For this review, take the finished solid that the model builds, in its own axes (mm). Face numbers are marked on the shaded views. A direction names the side the tool comes from. Coordinates: 2 decimals unless noted, no trailing zeros. Loops run counter-clockwise (first coordinate to the right, second up) from the corner with the lowest first, then second, coordinate; pieces in that order, holes last. Notation, with made-up numbers: (80, 83.5) - (85, 83.5) arc R30 ccw to (85, 118.5) - close; hole circle Ø2 at (47, 61). An arc over 180 degrees is marked (long way). Answer as a JSON object with one key per item and string values. Group by question number.
Item 1: We need section D-D (y = 0.5). Give the boundary of the cut face in (x, z).
Item 2: We need section A-A (y = -12). Give the boundary of the cut face in (x, z).
Item 3: We need section B-B (x = 30.5). Give the boundary of the cut face in (y, z), then the cut area to 3 significant figures.
Item 4: To check wall thickness, follow line 1 (Z direction, x = 13, y = 0.75); line 2 (X direction, y = 0, z = 18); line 3 (Y direction, x = 2, z = 17.5). State the ranges of each line that lie inside material, in increasing order.
Item 5: We need section C-C (z = 24.5). Give the boundary of the cut face in (x, y), then the cut area to 3 significant figures.
Item 6: Clearance check with flat-ended pins moving along their axes: pin 1 (2.5 mm diameter, centred on x = 10.5, z = 1.5, fed in from -Y); pin 2 (1 mm diameter, centred on x = 0, y = 0, fed in from +Z); pin 3 (2.5 mm diameter, centred on y = -6.5, z = 1.5, fed in from -X). State where each tip first meets the part, or that it passes through.
Item 7: Tool access review of the marked faces 1 and 2: name each direction out of +Z, -Z, +X, -X, +Y, -Y from which nothing blocks a thin tool from reaching the whole face with its end or side.
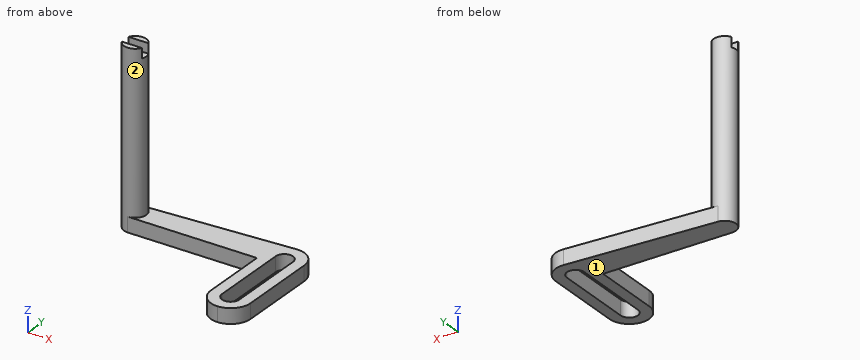
from build123d import *

# Parameters (mm, degrees)
EXTRUDE_1_DEPTH     = 3
SKETCH_1_3_R        = 2.25
EXTRUDE_2_DEPTH     = 35
SKETCH_2_W          = 5
SKETCH_2_H          = 2
CUT_EXTRUDE_1_DEPTH = 2
FILLET_1_R          = 4


with BuildPart() as part:
    # 草图1 → 凸台-拉伸1 (new body)
    with BuildSketch(Plane.XY):
        with BuildLine():
            Line((29.766666667, 3.993188645), (-0.13125, 2.246168613))
            ThreePointArc((-0.13125, 2.246168613), (-2.249041949, -0.065652955), (0, -2.25))
            Line((0, -2.25), (26, -2.25))
            Line((26, -2.25), (26, -20))
            Line((26, -20), (34, -20))
            Line((34, -20), (34, 0))
            ThreePointArc((34, 0), (32.744691847, 2.909753712), (29.766666667, 3.993188645))
        make_face()
        with BuildLine():
            Line((28.25, -16), (28.25, 0))
            ThreePointArc((28.25, 0), (30, 1.75), (31.75, 0))
            Line((31.75, 0), (31.75, -16))
            ThreePointArc((31.75, -16), (30, -17.75), (28.25, -16))
        make_face(mode=Mode.SUBTRACT)
    extrude(amount=EXTRUDE_1_DEPTH)

    # 草图1<3> → 凸台-拉伸2 (add)
    with BuildSketch(Plane.XY):
        with Locations(Location((0, 0, 0), (0, 0, 93.344152204))):
            Circle(SKETCH_1_3_R)
    extrude(amount=EXTRUDE_2_DEPTH)

    # 草图2 → 切除-拉伸1 (cut)
    with BuildSketch(Plane.XY.offset(35)):
        Rectangle(SKETCH_2_W, SKETCH_2_H)
    extrude(amount=-CUT_EXTRUDE_1_DEPTH, mode=Mode.SUBTRACT)

    # 圆角1
    fillet_1_edges = [part.edges().sort_by_distance(p)[0] for p in [
        (26, -20, 1.5),
        (34, -20, 1.5),
    ]]
    fillet(fillet_1_edges, radius=FILLET_1_R - 0.0001)  # a hair under: the kernel refuses the full size


solid = part.part
Check sheet entries:
{
 "1": {"outline": "(-2.19, 0) - (28.32, 0) - (28.32, 3) - (2.19, 3) - (2.19, 33) - (-2.19, 33) - close; (31.68, 0) - (33.97, 0) - (33.97, 3) - (31.68, 3) - close"},
 "2": {"outline": "(26, 0) - (28.25, 0) - (28.25, 3) - (26, 3) - close; (31.75, 0) - (34, 0) - (34, 3) - (31.75, 3) - close"},
 "3": {"outline": "(-19.97, 0) - (-17.68, 0) - (-17.68, 3) - (-19.97, 3) - close; (1.68, 0) - (3.97, 0) - (3.97, 3) - (1.68, 3) - close", "area": "13.7 mm2"},
 "4": {"line 1": "z = 0 to 3", "line 2": "x = -2.25 to 2.25", "line 3": "y = -1.03 to 1.03"},
 "5": {"outline": "circle Ø4.5 at (0, 0)", "area": "15.9 mm2"},
 "6": {"pin 1": "stops at y = -2.25", "pin 2": "stops at z = 33", "pin 3": "stops at x = 26"},
 "7": {"face 1": "-Z, +X, -X, +Y, -Y", "face 2": "+Z"}
}
